Autodesk Fusion 360 part; units mm, degrees
sketch "Sketch1" plane through (0, 0, 0) normal (0, 0, 1) x (1, 0, 0)
  circle A0 centre (0, 0) radius 48.5
  circle A1 centre (0, 0) radius 44.15
  circle A2 centre (0, 0) radius 42.15
  circle A3 centre (0, 0) radius 24
  line L0 (-4, 0) -> (4, 0)
  line L1 (4, 0) -> (4, 46)
  line L2 (4, 46) -> (-4, 46)
  line L3 (-4, 46) -> (-4, 0)
  line L4 (-2, 3.4641) -> (-41.8372, -19.5359)
  line L5 (-41.8372, -19.5359) -> (-37.8372, -26.4641)
  line L6 (-37.8372, -26.4641) -> (2, -3.4641)
  line L7 (2, -3.4641) -> (-2, 3.4641)
  line L8 (-2, -3.4641) -> (37.8372, -26.4641)
  line L9 (37.8372, -26.4641) -> (41.8372, -19.5359)
  line L10 (41.8372, -19.5359) -> (2, 3.4641)
  line L11 (2, 3.4641) -> (-2, -3.4641)
  circle A4 centre (0, 0) radius 6
  line L12 (15, 15) -> (-15, 15)
  line L13 (-15, 15) -> (-15, -15)
  line L14 (-15, -15) -> (15, -15)
  line L15 (15, -15) -> (15, 15)
  line L16 (15, 15) -> (-15, -15) construction
  line L17 (-15, 15) -> (15, -15) construction
  dimension "d1" = 97
  dimension "d2" = 88.3
  dimension "d3" = 84.3
  dimension "d4" = 48
  dimension "d6" = 360
  dimension "d7" = 12
  dimension "d12" = 30
  dimension "d13" = 30
extrude "Extrude1" add sketch "Sketch1" along normal blind 6 contours A0 | A1 L1 L2 L3 | A1 L8 L9 L10 | A2 A3 L1 L3 | A2 A3 L8 L10 | A1 L4 L5 L6 | A2 A3 L4 L6 | L1 L10 A4 L12 L15 | L1 L3 A4 L12 | L8 L10 A4 L15 | L3 L4 A4 L12 L13 | L6 L8 A4 L13 L14 L15 | L4 L6 A4 L13 makes body 1 at (48.4397, -2.4175, 4) makes body 2 at (-3.113, 29.8622, 0) makes body 3 at (-0.1495, 11.9944, 0) makes body 4 at (-27.4179, -12.2352, 0) makes body 5 at (27.4179, -12.2352, 0)
extrude "Extrude6" add sketch "Sketch1" along normal blind 6 contours A3 L1 L3 L12 | A3 L1 L10 L12 L15 | A3 L8 L10 L15 | A3 L3 L4 L12 L13 | A3 L6 L8 L13 L14 L15 | A3 L4 L6 L13 bodies 3 4 2 5
sketch "Sketch2" plane through (0, 0, 0) normal (0, 0, 1) x (1, 0, 0)
extrude "Extrude2" add sketch "Sketch1" along normal blind 65 contours A1 A2 L1 L10 | A1 A2 L1 L3 | A1 A2 L8 L10 | A1 A2 L3 L4 | A1 A2 L6 L8 | A1 A2 L4 L6 bodies 1 3
sketch "Sketch4" plane through (0, 0, 65) normal (0, 0, 1) x (-1, 0, 0)
  circle A0 centre (0, 0) radius 42.15
  circle A1 centre (0, 0) radius 44.15
  line L0 (-3.9193, -45.9529) -> (3.9193, -45.9529)
  line L1 (3.9193, -45.9529) -> (3.9193, 45.9529)
  line L2 (3.9193, 45.9529) -> (-3.9193, 45.9529)
  line L3 (-3.9193, 45.9529) -> (-3.9193, -45.9529)
  line L4 (-3.9193, -45.9529) -> (3.9193, 45.9529) construction
  line L5 (3.9193, -45.9529) -> (-3.9193, 45.9529) construction
  line L6 (41.7561, 19.5823) -> (37.8368, 26.3707)
  line L7 (-37.8368, -26.3707) -> (41.7561, 19.5823)
  line L8 (37.8368, 26.3707) -> (-41.7561, -19.5823)
  line L9 (-41.7561, -19.5823) -> (-37.8368, -26.3707)
  line L10 (-37.8368, 26.3707) -> (-41.7561, 19.5823)
  line L11 (41.7561, -19.5823) -> (-37.8368, 26.3707)
  line L12 (-41.7561, 19.5823) -> (37.8368, -26.3707)
  line L13 (37.8368, -26.3707) -> (41.7561, -19.5823)
  circle A2 centre (0, 0) radius 6
  circle A3 centre (0, 0) radius 24
  line L14 (-15, 15) -> (15, 15)
  line L15 (15, 15) -> (15, -15)
  line L16 (15, -15) -> (-15, -15)
  line L17 (-15, -15) -> (-15, 15)
  line L18 (-15, 15) -> (15, -15) construction
  line L19 (15, 15) -> (-15, -15) construction
  dimension "d20" = 360
  dimension "d21" = 12
  dimension "d22" = 48
  dimension "d25" = 30
  dimension "d26" = 30
extrude "Extrude4" add sketch "Sketch4" against normal blind 6 contours A0 L7 L8 A3 | L7 L11 A3 L15 | L7 L8 A3 L15 | L11 L12 A3 L15 | L1 L8 A3 L14 L15 | A0 L1 L3 A3 | L1 L12 A3 L15 L16 | L1 L3 A3 L14 | L1 L3 A3 L16 | A0 L11 L12 A3 | L3 L11 A3 L14 L17 | L3 L7 A3 L16 L17 | L11 L12 A3 L17 | L7 L8 A3 L17 | L8 L12 A3 L17 picked at (24.3429, 17.5763) picked at (3.0501, -29.8698) picked at (-27.393, 12.2934) bodies 1
sketch "Sketch5" plane through (0, 0, 65) normal (0, 0, 1) x (-1, 0, 0)
  arc A0 (3.9193, -41.9674) -> (38.3045, 17.5895) centre (0, 0) ccw
  line L0 (3.9193, -41.9674) -> (3.9193, -23.6778)
  arc A1 (3.9193, -23.6778) -> (22.4652, 8.4447) centre (0, 0) ccw
  line L1 (22.4652, 8.4447) -> (38.3045, 17.5895)
  line L2 (34.3852, 24.3779) -> (18.5459, 15.2331)
  line L3 (-18.5459, 15.2331) -> (-34.3852, 24.3779)
  arc A2 (34.3852, 24.3779) -> (-34.3852, 24.3779) centre (0, 0) ccw
  line L4 (-38.3045, 17.5895) -> (-22.4652, 8.4447)
  arc A3 (-22.4652, 8.4447) -> (-3.9193, -23.6778) centre (0, 0) ccw
  line L5 (-3.9193, -23.6778) -> (-3.9193, -41.9674)
  arc A4 (-38.3045, 17.5895) -> (-3.9193, -41.9674) centre (0, 0) ccw
  circle A5 centre (0, 0) radius 44.15
  arc A6 (18.5459, 15.2331) -> (-18.5459, 15.2331) centre (0, 0) ccw
  line L6 (15, -15) -> (-15, -15)
  line L7 (-15, -15) -> (-15, 15)
  line L8 (-15, 15) -> (15, 15)
  line L9 (15, 15) -> (15, -15)
extrude "Extrude5" add sketch "Sketch4" against normal blind 3 contours L7 L11 L15 | L1 L7 L8 L11 A2 L15 | L1 L7 L11 L12 A2 L15 | L1 L8 L14 L15 | L7 L11 A2 | L1 L12 L15 L16 | L1 L3 L8 L11 A2 L14 | L1 L8 A2 | L1 L3 L7 L12 A2 L16 | L1 L12 A2 | L3 L11 L14 L17 | L3 L7 L16 L17 | L3 L8 L11 L12 A2 L17 | L3 L11 A2 | L3 L7 L8 L12 A2 L17 | L3 L7 A2 | L8 L12 L17 | L8 L12 A2 bodies 1
extrude "Extrude7" add sketch "Sketch4" against normal blind 6 contours L7 L11 L15 | L1 L7 L8 L11 A2 L15 | L1 L7 L11 L12 A2 L15 | L1 L8 L14 L15 | L7 L11 A2 | L1 L12 L15 L16 | L1 L3 L8 L11 A2 L14 | L1 L8 A2 | L1 L3 L7 L12 A2 L16 | L1 L12 A2 | L3 L11 L14 L17 | L3 L7 L16 L17 | L3 L8 L11 L12 A2 L17 | L3 L11 A2 | L3 L7 L8 L12 A2 L17 | L3 L7 A2 | L8 L12 L17 | L8 L12 A2 bodies 1
sketch "Sketch8" plane through (0, 0, 0) normal (0, 0, 1) x (1, 0, 0)
sketch "Sketch9" plane through (0, 0, 0) normal (0, 0, 1) x (1, 0, 0)
  line L0 (10, 10) -> (-10, 10)
  line L1 (-10, 10) -> (-10, -10)
  line L2 (-10, -10) -> (10, -10)
  line L3 (10, -10) -> (10, 10)
  line L4 (10, 10) -> (-10, -10) construction
  line L5 (-10, 10) -> (10, -10) construction
  dimension "d33" = 20
sketch "Sketch10" plane through (0, 0, 0) normal (0, 0, 1) x (1, 0, 0)
sketch "Sketch13" plane through (0, 0, 0) normal (0, 0, -1) x (1, 0, 0)
  arc A0 (4, -41.9598) -> (38.3382, 17.5158) centre (0, 0) ccw
  line L0 (4, -41.9598) -> (4, -23.6643)
  arc A1 (4, -23.6643) -> (22.4939, 8.3681) centre (0, 0) ccw
  line L1 (22.4939, 8.3681) -> (38.3382, 17.5158)
  arc A2 (-38.3382, 17.5158) -> (-4, -41.9598) centre (0, 0) ccw
  line L2 (-38.3382, 17.5158) -> (-22.4939, 8.3681)
  arc A3 (-22.4939, 8.3681) -> (-4, -23.6643) centre (0, 0) ccw
  line L3 (-4, -23.6643) -> (-4, -41.9598)
  circle A4 centre (0, 0) radius 6
  line L4 (34.3382, 24.444) -> (18.4939, 15.2963)
  arc A5 (18.4939, 15.2963) -> (-18.4939, 15.2963) centre (0, 0) ccw
  line L5 (-18.4939, 15.2963) -> (-34.3382, 24.444)
  arc A6 (34.3382, 24.444) -> (-34.3382, 24.444) centre (0, 0) ccw
  circle A7 centre (0, 0) radius 48.5
sketch "Sketch14" plane through (0, 0, 0) normal (0, 0, -1) x (1, 0, 0)
  line L0 (0, 0) -> (0, 210)
  line L1 (0, 210) -> (47.0531, 2.6393)
  line L2 (47.0531, 2.6393) -> (-47.1343, 2.6393)
  line L3 (-47.1343, 2.6393) -> (0, 210)
  dimension "d54" = 210
extrude "Extrude8" add sketch "Sketch14" against normal blind 6 bodies 1
fillet "Fillet1" radius 13 1 edges at (0, -210, 3) on bodies 1
extrude "Extrude9" cut sketch "Sketch9" sketch "Sketch1" along normal blind 2 of sketch 2 contours L1 L10 A4 L12 L15 | L1 L3 A4 L12 | L8 L10 A4 L15 | L3 L4 A4 L12 L13 | L6 L8 A4 L13 L14 L15 | L4 L6 A4 L13 bodies 1
extrude "Extrude10" cut sketch "Sketch13" against normal blind 11 contours A4 bodies 1
sketch "Sketch15" plane through (0, 0, 0) normal (0, 0, -1) x (1, 0, 0)
  line L0 (-15, 15) -> (15, 15)
  line L1 (15, 15) -> (15, -15)
  line L2 (15, -15) -> (-15, -15)
  line L3 (-15, -15) -> (-15, 15)
  arc A0 (12.6668, 154.1781) -> (-12.6876, 154.1828) centre (-0.0109, 151.3013) ccw
  line L4 (-12.6876, 154.1828) -> (-42.3691, 23.6032)
  arc A1 (-42.3691, 23.6032) -> (42.2464, 23.8222) centre (0, 0) ccw
  line L5 (42.2464, 23.8222) -> (12.6668, 154.1781)
  arc A2 (-23.8544, 2.6393) -> (-4, -23.6643) centre (0, 0) ccw
  line L6 (-4, -23.6643) -> (-4, -41.9598)
  arc A3 (-42.0673, 2.6393) -> (-4, -41.9598) centre (0, 0) ccw
  line L7 (-42.0673, 2.6393) -> (-23.8544, 2.6393)
  line L8 (23.8544, 2.6393) -> (42.0673, 2.6393)
  arc A4 (4, -41.9598) -> (42.0673, 2.6393) centre (0, 0) ccw
  line L9 (4, -41.9598) -> (4, -23.6643)
  arc A5 (4, -23.6643) -> (23.8544, 2.6393) centre (0, 0) ccw
sketch "Sketch16" plane through (0, 0, 6) normal (0, 0, 1) x (-1, 0, 0)
  arc A0 (12.6876, 154.1828) -> (-12.6668, 154.1781) centre (0.0109, 151.3013) ccw
  line L0 (-12.6668, 154.1781) -> (-42.2464, 23.8222)
  arc A1 (-42.2464, 23.8222) -> (42.3691, 23.6032) centre (0, 0) ccw
  line L1 (42.3691, 23.6032) -> (12.6876, 154.1828)
  circle A2 centre (0, 0) radius 44.15
  circle A3 centre (0.0109, 151.3013) radius 7.5884
extrude "Extrude11" add sketch "Sketch16" along normal blind 7 draft 40 contours A3 bodies 1
hole "Hole7" at (-0.0109, -151.3013, 0) direction (0, 0, 1) diameter 7.05 depth 22 tip angle 180 bodies 1
Source: CAD feature listing. Evaluate the final solid. Frame: model axes, mm. A direction names the side the tool comes from. Coordinates: 2 decimals unless noted, no trailing zeros. Loops run counter-clockwise (first coordinate to the right, second up) from the corner with the lowest first, then second, coordinate; pieces in that order, holes last. Notation, with made-up numbers: M 54,7 L 98,7 A16 ccw 98,14 Z; hole C 13.5,-20.5 d6. An arc over 180 degrees is marked long. Use a Markdown table: item, result. Add a question column.
Q1. Section query C-C, the plane z = 51.5. Return loops of the section in (x, y).
Q2. Material intervals for L1, parallel to X at y = 0, z = 3; L2, parallel to X at y = 0, z = 63; L3, parallel to Y at x = 0, z = 14.5, sorted ascending.
Q3. Draft query along Y for faces 6 (the flat face through (-3, -148, 13)), 7 (the flat face through (27.25, -89.91, 2.96)), 8 (the flat face through (0.5, -6.4, 59)). Return one class per face: pulls with the +Y half, pulls with the -Y half, needs draft (parallel to the pull), parting line crosses it, or undercut.
Q4. First-contact query: pin 1 (12 mm diameter, centred on x = 11.5, z = 57, fed in from +Y); pin 2 (3 mm diameter, centred on x = -26.5, z = 44, fed in from -Y); pin 3 (5 mm diameter, centred on y = 28.5, z = 3.5, fed in from +X). Flat tips, straight axial feed; report the tip coordinate or a pass-through.
Q5. Section query B-B, the plane y = 0. State how many separate pieces and enclosed holes the cut face has, and give its area (3 significant figures).
Q6. Section query A-A, the plane x = 29. Return loops of the section in (y, z), and give its area (3 significant figures).
Q7. Access query for faces 1 (the cylindrical face through (-19.308, 14.255, 2.958)), 2 (the flat face through (-30.27, -12.95, 62.04)), 3 (the cylindrical face through (-0.3, -164.3, 3)), 4 (the flat face through (-7, 0, 2)), 5 (the conical face through (1.71, -143.53, 6.44)). Directions: +Z, -Z, +X, -X, +Y, -Y. A direction counts if a zero-diameter tool reaches every point of the face in a straight line with its end or side. Return the directions, or none.
Result:
| question | item | result |
|---|---|---|
| 1 | outline | C 0,0 d88.3; hole C 0,0 d84.3 |
| 2 | L1 | x = -48.5 to -42.15, -24 to -6, 6 to 24, 42.15 to 48.5 |
| 2 | L2 | x = -44.15 to -42.15, -24 to -6, 6 to 24, 42.15 to 44.15 |
| 2 | L3 | y = -44.15 to -42.15, 42.15 to 44.15 |
| 3 | face 6 | needs draft |
| 3 | face 7 | pulls with the -Y half |
| 3 | face 8 | undercut |
| 4 | pin 1 | stops at y = 43.81 |
| 4 | pin 2 | stops at y = -36.39 |
| 4 | pin 3 | stops at x = 40.94 |
| 5 | separate pieces | 6 |
| 5 | enclosed holes | 0 |
| 5 | area | 708 mm2 |
| 6 | outline | M -82.2,0 L -2.64,0 L -2.64,6 L -30.59,6 L -30.59,65 L -33.29,65 L -33.29,6 L -82.2,6 Z; M -21.27,59 L -12.22,59 L -12.22,65 L -21.27,65 Z; M 30.59,0 L 38.87,0 L 38.87,6 L 33.29,6 L 33.29,65 L 30.59,65 Z |
| 6 | area | 900 mm2 |
| 7 | face 1 | +Z, -Z |
| 7 | face 2 | +Z |
| 7 | face 3 | -Z, -Y |
| 7 | face 4 | -Z |
| 7 | face 5 | none |
